Autodesk Inventor part; units mm, degrees
ref_plane "YZ Plane" through (0, 0, 0) normal (1, 0, 0) x (0, 1, 0)
ref_plane "XZ Plane" through (0, 0, 0) normal (0, 1, 0) x (-1, 0, 0)
ref_plane "XY Plane" through (0, 0, 0) normal (0, 0, 1) x (1, 0, 0)
sketch "Sketch1" plane through (0, 0, 0) normal (1, 0, 0) x (0, 1, 0)
  line L0 (1.91, 21.4) -> (-1.91, 21.4)
  line L1 (-1.91, 21.4) -> (-1.91, 30.1)
  line L2 (-1.91, 30.1) -> (1.91, 30.1)
  line L3 (1.91, 21.4) -> (1.91, 0)
  line L4 (1.91, 30.1) -> (1.91, 35.1)
  line L5 (1.91, 35.1) -> (-5.59, 35.1)
  line L6 (-5.59, 35.1) -> (-5.59, 0)
  line L7 (-5.59, 0) -> (1.91, 0)
  point P0 (0, 0)
  dimension "d4" = 5
  dimension "d5" = 7.5
revolve "Revolution1" add sketch "Sketch1" angle 360 about axis through (0, -5.59, 0) along (0, 1, 0)
chamfer "Chamfer1" distance 1.5 angle 45 2 edges at (0, 1.91, -30.1) (0, 1.91, -21.4)
move faces "Move1" translate (0, 1.5, 0) faces at (6.585, 1.91, -0.7996) (-3.3526, 0.91, 20.6294) (-2.5025, 1.41, 30.9992) (3.8791, 1.91, -32.3815)
ref_plane "Work Plane1" through (0, 6.29, 0) normal (0, 1, 0) x (1, 0, 0)
properties part number "Spinner_Base"
Design review of the part built by this model. Coordinates are the model's own, in mm. A direction names the side the tool comes from. Round coordinates to 2 decimals unless told otherwise and drop trailing zeros. Write each loop counter-clockwise with the first axis right and the second up, starting at its lowest first coordinate (ties: lowest second). Pieces come first, ordered by that corner, then holes. Notation, with made-up numbers: (81, -15.5) - (116, -15.5) arc R8 ccw to (116, -4.5) - close; hole circle Ø3 at (29, 44.25). An arc over 180 degrees is marked (long way). Return JSON: item names as keys, results as strings. Group by question number.
Item 1: For probe 1 along Z at (x, y) = (2, 0.25); probe 2 along X at (y, z) = (2, -3.5); probe 3 along X at (y, z) = (2, 17), list the stretches that pass through material, from the lowest coordinate up. Write a range as [from, to].
Item 2: Insertion check: P1, Ø4, axis at y = 2, z = -23, coming from the +X side; P2, Ø12, axis at x = -23.5, z = 27, coming from the -Y side; P3, Ø1.5, axis at y = -3, z = -23.5, coming from the -X side; P4, Ø1.5, axis at y = 1.5, z = 21, coming from the +X side. Each pin has a flat end and moves straight along its axis. Give the tip position at first contact, or say it passes through.
Item 3: The part is to be moulded in two halves that separate along Z. For faces 3 (the face through (21.36, -1.15, -27.85)), 4 (the face through (0, -5.59, 0)), 5 (the face through (-29.384, 0.027, -6.525)), say which applies: pulls with the +Z half, pulls with the -Z half, needs draft (parallel to the pull), parting line crosses it, or undercut.
Item 4: Machinability: for faces 1 (the face through (20.5, -1.91, -7.1)), 2 (the face through (0, 3.41, 0)), which of the approach directions +Z, -Z, +X, -X, +Y, -Y give a long, thin tool a straight path to every point of the face, cutting with its end or side? Answer none if there is none.
Item 5: We need section C-C on x = 0. Write out the cut boundary in (y, z).
Item 6: We need section B-B on z = 0. Write out the cut boundary in (x, y).
Item 7: We need section D-D on y = -3.75. Write out the cut boundary in (x, z), and give its area (3 significant figures).
Item 8: We need section A-A on y = -0.25. Write out the cut boundary in (x, z).
Model answer:
{
 "1": {"probe 1": "z = [-35.04, -30.03], [-21.31, 21.31], [30.03, 35.04]", "probe 2": "x = [-34.93, -29.99], [-21.02, 21.02], [29.99, 34.93]", "probe 3": "x = [-30.71, -24.95], [-12.85, 12.85], [24.95, 30.71]"},
 "2": {"P1": "stops at x = 28.12", "P2": "stops at y = -5.59", "P3": "stops at x = -26.73", "P4": "stops at x = 28.67"},
 "3": {"face 3": "parting line crosses it", "face 4": "needs draft", "face 5": "undercut"},
 "4": {"face 1": "+Y", "face 2": "+Z, -Z, +X, -X, +Y"},
 "5": {"outline": "(-5.59, -35.1) - (3.41, -35.1) - (3.41, -31.6) - (1.91, -30.1) - (-1.91, -30.1) - (-1.91, -21.4) - (1.91, -21.4) - (3.41, -19.9) - (3.41, 19.9) - (1.91, 21.4) - (-1.91, 21.4) - (-1.91, 30.1) - (1.91, 30.1) - (3.41, 31.6) - (3.41, 35.1) - (-5.59, 35.1) - close"},
 "6": {"outline": "(-35.1, -5.59) - (35.1, -5.59) - (35.1, 3.41) - (31.6, 3.41) - (30.1, 1.91) - (30.1, -1.91) - (21.4, -1.91) - (21.4, 1.91) - (19.9, 3.41) - (-19.9, 3.41) - (-21.4, 1.91) - (-21.4, -1.91) - (-30.1, -1.91) - (-30.1, 1.91) - (-31.6, 3.41) - (-35.1, 3.41) - close"},
 "7": {"outline": "circle Ø70.2 at (0, 0)", "area": "3,870 mm²"},
 "8": {"outline": "circle Ø70.2 at (0, 0); circle Ø42.8 at (0, 0); hole circle Ø60.2 at (0, 0)"}
}
